Verification items for the finished model (mm, model axes). A direction names the side the tool comes from. Coordinates: 2 decimals unless noted, no trailing zeros. Loops run counter-clockwise (first coordinate to the right, second up) from the corner with the lowest first, then second, coordinate; pieces in that order, holes last. Notation, with made-up numbers: (1, 89) -> (26, 89) arc R14 cw to (26, 111) -> close; hole circle Ø5 at (84, 45). An arc over 180 degrees is marked (long way). Answer as a JSON object with one key per item and string values. Group by question number.
Q1. Cross-section at B-B on y = 10. Record the boundary of the cut face in (x, z), and give its area (3 significant figures).
Q2. Cross-section at A-A on x = 0. Record the boundary of the cut face in (y, z), and give its area (3 significant figures).
Q3. Set-up check for faces 1 (the flat face through (0, 21, 3)), 2 (the cylindrical face through (0, 7, 2)): record each of +Z, -Z, +X, -X, +Y, -Y from which the full face is reachable in a straight line by a thin tool's end or side.
Q4. Cross-section at D-D on z = 4.9. Record the boundary of the cut face in (x, y), and give its area (3 significant figures).
Q5. Cross-section at C-C on y = 18. Record the boundary of the cut face in (x, z).
Q6. Scan lines: L1, parallel to Y at x = 0, z = 1.1; L2, parallel to X at y = -10, z = 5.3; L3, parallel to Y at x = -1, z = 3. Record each from-to range of solid material in increasing order.
Q7. Gauge pin test, flat ends, axial feed: pin 1 Ø3 at (y, z) = (10, 5) entering from -X; pin 2 Ø3 at (x, y) = (-1, -10.5) entering from -Z; pin 3 Ø1.8 at (x, y) = (0, -10) entering from +Z. Record the tip position at first contact, or that the pin passes through.
Q8. Release check for a two-part mould opening along Y. For faces 3 (the flat face through (0, -21, 3)), 4 (the flat face through (1.3, -8.7, 3.5)), 5 (the flat face through (17, 0, 3)) record: released by +Y, released by -Y, zero draft, split by the parting line, or undercut.
```python
from build123d import *

# Parameters (mm, degrees)
F0_W     = 38
F0_H     = 42
F1_DEPTH = 6
F3_DEPTH = 42
F4_R     = 0.5
F5_R     = 3
F6_DEPTH = 3.5
F7_R     = 1.5
F8_R     = 1.5
F9_DEPTH = 5


with BuildPart() as f1:
    # F0 (on Top) → F1 (new body)
    with BuildSketch(Plane.XY):
        Rectangle(F0_W, F0_H)
    extrude(amount=F1_DEPTH)

    # F2 (on face) → F3 (cut)
    with BuildSketch(Plane.XZ.offset(21)):
        Polygon((15, 6), (19, 0), (19, 6), align=None)
        Polygon((-15, 6), (-19, 6), (-19, 0), align=None)
    extrude(amount=-F3_DEPTH, mode=Mode.SUBTRACT)

    # F4
    f4_edges = [f1.edges().sort_by_distance(p)[0] for p in [
        (-19, 0, 0),
        (19, 0, 0),
        (-15, 0, 6),
        (15, 0, 6),
    ]]
    fillet(f4_edges, radius=F4_R)

    # F5 (on face) → F6 (cut)
    with BuildSketch(Plane(origin=(0, 0, 0), x_dir=(1, 0, 0), z_dir=(0, 0, -1))):
        with Locations((0, 10)):
            Circle(F5_R)
        with Locations((0, -10)):
            Circle(F5_R)
    extrude(amount=-F6_DEPTH, mode=Mode.SUBTRACT)

    # F7 (on face) + F8 (on face) → F9 (cut)
    with BuildSketch(Plane(origin=(0, 0, 3.5), x_dir=(1, 0, 0), z_dir=(0, 0, -1))):
        with Locations((0, 10)):
            Circle(F7_R)
    with BuildSketch(Plane(origin=(0, 0, 3.5), x_dir=(1, 0, 0), z_dir=(0, 0, -1))):
        with Locations((0, -10)):
            Circle(F8_R)
    extrude(amount=-F9_DEPTH, mode=Mode.SUBTRACT)


solid = f1.part
```
Computed values:
{
 "1": {"outline": "(-18.48, 0.78) arc R0.5 ccw to (-18.07, 0) -> (-3, 0) -> (-3, 3.5) -> (-1.5, 3.5) -> (-1.5, 6) -> (-14.73, 6) arc R0.5 ccw to (-15.15, 5.78) -> close; (1.5, 3.5) -> (3, 3.5) -> (3, 0) -> (18.07, 0) arc R0.5 ccw to (18.48, 0.78) -> (15.15, 5.78) arc R0.5 ccw to (14.73, 6) -> (1.5, 6) -> close", "area": "175 mm²"},
 "2": {"outline": "(-21, 0) -> (-13, 0) -> (-13, 3.5) -> (-11.5, 3.5) -> (-11.5, 6) -> (-21, 6) -> close; (-8.5, 3.5) -> (-7, 3.5) -> (-7, 0) -> (7, 0) -> (7, 3.5) -> (8.5, 3.5) -> (8.5, 6) -> (-8.5, 6) -> close; (11.5, 3.5) -> (13, 3.5) -> (13, 0) -> (21, 0) -> (21, 6) -> (11.5, 6) -> close", "area": "195 mm²"},
 "3": {"face 1": "+Z, -Z, +X, -X, +Y", "face 2": "-Z"},
 "4": {"outline": "(-15.73, -21) -> (15.73, -21) -> (15.73, 21) -> (-15.73, 21) -> close; hole circle Ø3 at (0, -10); hole circle Ø3 at (0, 10)", "area": "1,310 mm²"},
 "5": {"outline": "(-18.48, 0.78) arc R0.5 ccw to (-18.07, 0) -> (18.07, 0) arc R0.5 ccw to (18.48, 0.78) -> (15.15, 5.78) arc R0.5 ccw to (14.73, 6) -> (-14.73, 6) arc R0.5 ccw to (-15.15, 5.78) -> close"},
 "6": {"L1": "y = -21 to -13, -7 to 7, 13 to 21", "L2": "x = -15.47 to -1.5, 1.5 to 15.47", "L3": "y = -21 to -12.83, -7.17 to 7.17, 12.83 to 21"},
 "7": {"pin 1": "stops at x = -16.67", "pin 2": "stops at z = 3.5", "pin 3": "passes through"},
 "8": {"face 3": "released by -Y", "face 4": "undercut", "face 5": "zero draft"}
}
